from build123d import *

# Parameters (mm, degrees)
SKETCH_1_W          = 72
SKETCH_1_H          = 72
SKETCH_1_R          = 13.5
EXTRUDE_1_DEPTH     = 4
SKETCH_2_R          = 1.65
CUT_EXTRUDE_5_DEPTH = 4
FILLET_1_R          = 2
SKETCH_3_W          = 3.5
SKETCH_3_H          = 55
SKETCH_3_W_2        = 55
SKETCH_3_H_2        = 3.5
EXTRUDE_2_DEPTH     = 3
FILLET_2_R          = 2


with BuildPart() as part:
    # 草图1 → 凸台-拉伸1 (new body)
    with BuildSketch(Plane(origin=(0, 0, 0), x_dir=(1, 0, 0), z_dir=(0, 1, 0))):
        Rectangle(SKETCH_1_W, SKETCH_1_H)
        with Locations(Location((0, 0, 0), (0, 0, 270))):
            Circle(SKETCH_1_R, mode=Mode.SUBTRACT)
    extrude(amount=EXTRUDE_1_DEPTH)

    # 草图2 → 切除-拉伸5 (cut)
    with BuildSketch(Plane(origin=(0, 0, 0), x_dir=(1, 0, 0), z_dir=(0, 1, 0))):
        with Locations(Location((-22, 22, 0), (0, 0, 270))):
            Circle(SKETCH_2_R)
        with Locations(Location((22, 22, 0), (0, 0, 270))):
            Circle(SKETCH_2_R)
        with Locations(Location((22, -22, 0), (0, 0, 270))):
            Circle(SKETCH_2_R)
        with Locations(Location((-22, -22, 0), (0, 0, 270))):
            Circle(SKETCH_2_R)
        with Locations(Location((-32.5, 32.5, 0), (0, 0, 270))):
            Circle(SKETCH_2_R)
        with Locations(Location((32.5, 32.5, 0), (0, 0, 270))):
            Circle(SKETCH_2_R)
        with Locations(Location((32.5, -32.5, 0), (0, 0, 270))):
            Circle(SKETCH_2_R)
        with Locations(Location((-32.5, -32.5, 0), (0, 0, 270))):
            Circle(SKETCH_2_R)
    extrude(amount=CUT_EXTRUDE_5_DEPTH, mode=Mode.SUBTRACT)

    # 圆角1
    fillet_1_edges = [part.edges().sort_by_distance(p)[0] for p in [
        (36, 2, 36),
        (-36, 2, 36),
        (-36, 2, -36),
        (36, 2, -36),
    ]]
    fillet(fillet_1_edges, radius=FILLET_1_R)

    # 草图3 → 凸台-拉伸2 (add)
    with BuildSketch(Plane(origin=(0, 4, 0), x_dir=(1, 0, 0), z_dir=(0, 1, 0))):
        with Locations((-34.25, 0)):
            Rectangle(SKETCH_3_W, SKETCH_3_H)
        with Locations((0, 34.25)):
            Rectangle(SKETCH_3_W_2, SKETCH_3_H_2)
        with Locations((34.25, 0)):
            Rectangle(SKETCH_3_W, SKETCH_3_H)
        with Locations((0, -34.25)):
            Rectangle(SKETCH_3_W_2, SKETCH_3_H_2)
    extrude(amount=EXTRUDE_2_DEPTH)

    # 圆角2
    fillet_2_edges = [part.edges().sort_by_distance(p)[0] for p in [
        (32.5, 4, 0),
        (0, 4, 32.5),
        (-32.5, 4, 0),
        (0, 4, -32.5),
    ]]
    fillet(fillet_2_edges, radius=FILLET_2_R)


solid = part.part
Verification items for the finished model (mm, model axes). A direction names the side the tool comes from. Round coordinates to 2 decimals unless told otherwise and drop trailing zeros. Write each loop counter-clockwise with the first axis right and the second up, starting at its lowest first coordinate (ties: lowest second). Pieces come first, ordered by that corner, then holes.
(1) Section check C-C (z = 22). Enter the section's corners in (x, y), plus the area to 3 significant figures.
Returned:
outline: (-36, 0) - (-23.65, 0) - (-23.65, 4) - (-30.5, 4) arc R2 cw to (-32.5, 6) - (-32.5, 7) - (-36, 7) - close; (-20.35, 0) - (20.35, 0) - (20.35, 4) - (-20.35, 4) - close; (23.65, 0) - (36, 0) - (36, 7) - (32.5, 7) - (32.5, 6) arc R2 cw to (30.5, 4) - (23.65, 4) - close
area: 284 mm2
(2) Material ranges on line 1 (X direction, y = 1.6, z = 32.5); line 2 (X direction, y = 2.7, z = 22); line 3 (X direction, y = 6.25, z = 19), recorded low to high.
Returned:
line 1: x = -36 to -34.15, -30.85 to 30.85, 34.15 to 36
line 2: x = -36 to -23.65, -20.35 to 20.35, 23.65 to 36
line 3: x = -36 to -32.5, 32.5 to 36
(3) Mould release check, pull along X, two halves, no side actions. Record for faces 1 (the cylindrical face through (31.9, 4.57, -0.39)), 2 (the cylindrical face through (-35.43, 2.03, -35.4)), 3 (the cylindrical face through (-30.864, 1.972, 32.285)), 4 (the flat face through (34, 5, -27.5)): pulls with the +X half, pulls with the -X half, needs draft (parallel to the pull), parting line crosses it, or undercut.
Returned:
face 1: undercut
face 2: pulls with the -X half
face 3: undercut
face 4: needs draft
(4) Section check B-B (x = 0). Enter the section's corners in (y, z).
Returned:
outline: (0, -36) - (7, -36) - (7, -32.5) - (6, -32.5) arc R2 cw to (4, -30.5) - (4, -13.5) - (0, -13.5) - close; (0, 13.5) - (4, 13.5) - (4, 30.5) arc R2 cw to (6, 32.5) - (7, 32.5) - (7, 36) - (0, 36) - close
(5) Access from +Z, -Z, +X, -X, +Y, -Y to the whole of each face (thin tool, end or side, straight path). Record for faces 5 (the cylindrical face through (23.115, 1.972, -23.216)), 6 (the flat face through (-27.5, 5, -34)), 7 (the flat face through (-34, 5, -27.5)), 8 (the cylindrical face through (0.39, 4.57, -31.9)), 9 (the flat face through (-34, 5, 27.5)).
Returned:
face 5: +Y, -Y
face 6: +Z, -Z, -X, +Y
face 7: -Z, +X, -X, +Y
face 8: +X, -X, +Y
face 9: +Z, +X, -X, +Y
(6) Depth check by flat-ended pin: pin 1 Ø0.9 at (x, y) = (-34, 6) entering from -Z; pin 2 Ø3 at (x, z) = (-22, -22) entering from -Y; pin 3 Ø0.9 at (y, z) = (5, -34) entering from +X; pin 4 Ø4 at (x, z) = (22, 22) entering from +Y. Enter the tip coordinate at first touch or a pass-through.
Returned:
pin 1: stops at z = -27.5
pin 2: passes through
pin 3: stops at x = 27.5
pin 4: stops at y = 4
(7) Section check D-D (y = 1). Give the number of separate pieces and of enclosed holes in the cut face, plus the area to 3 significant figures.
Returned:
separate pieces: 1
enclosed holes: 9
area: 4,540 mm2
(8) Section check A-A (x = 22). Enter the section's corners in (y, z).
Returned:
outline: (0, -36) - (7, -36) - (7, -32.5) - (6, -32.5) arc R2 cw to (4, -30.5) - (4, -23.65) - (0, -23.65) - close; (0, -20.35) - (4, -20.35) - (4, 20.35) - (0, 20.35) - close; (0, 23.65) - (4, 23.65) - (4, 30.5) arc R2 cw to (6, 32.5) - (7, 32.5) - (7, 36) - (0, 36) - close
